from build123d import *

# Parameters (mm, degrees)
SKETCH1_W            = 30
SKETCH1_H            = 105
BOSS_EXTRUDE1_DEPTH  = 4
SKETCH2_W            = 30
SKETCH2_H            = 12
SKETCH2_R            = 1.8
BOSS_EXTRUDE2_DEPTH  = 4
SKETCH3_W            = 7
SKETCH3_H            = 16
CUT_EXTRUDE1_DEPTH   = 110.494292089
BOSS_EXTRUDE3_DEPTH  = 4
BOSS_EXTRUDE4_START  = -30
BOSS_EXTRUDE4_DEPTH  = 4
SKETCH5_W            = 30
SKETCH5_H            = 41
BOSS_EXTRUDE5_DEPTH  = 4
SKETCH6_W            = 30
SKETCH6_H            = 135
BOSS_EXTRUDE6_DEPTH  = 4
SKETCH7_W            = 30
SKETCH7_H            = 8.5
BOSS_EXTRUDE7_DEPTH  = 4
FILLET1_R            = 1.1
SKETCH10_W           = 2.15
SKETCH10_H           = 4
SKETCH11_W           = 8
SKETCH11_H           = 8.5
CUT_EXTRUDE2_DEPTH   = 16
SKETCH14_W           = 1.8
SKETCH14_H           = 30
BOSS_EXTRUDE8_DEPTH  = 1
SKETCH16_W           = 3.4
SKETCH16_H           = 4
BOSS_EXTRUDE10_DEPTH = 1
BOSS_EXTRUDE9_START  = -30
BOSS_EXTRUDE9_DEPTH  = 1
SKETCH17_W           = 3.4
SKETCH17_H           = 4
BOSS_EXTRUDE11_DEPTH = 1
CHAMFER1_SIZE        = 3
FILLET2_R            = 2


with BuildPart() as part:
    # Sketch1 → Boss-Extrude1 (new body)
    with BuildSketch(Plane.XY):
        with Locations((15, 52.5)):
            Rectangle(SKETCH1_W, SKETCH1_H)
    extrude(amount=BOSS_EXTRUDE1_DEPTH)

    # Sketch2 → Boss-Extrude2 (add)
    with BuildSketch(Plane.XZ):
        with Locations((15, 6)):
            Rectangle(SKETCH2_W, SKETCH2_H)
        with Locations((15, 5)):
            Circle(SKETCH2_R, mode=Mode.SUBTRACT)
    extrude(amount=-BOSS_EXTRUDE2_DEPTH)

    # Sketch3 → Cut-Extrude1 (cut, through all)
    with BuildSketch(Plane.XY.offset(4)):
        with Locations((15, 12)):
            Rectangle(SKETCH3_W, SKETCH3_H)
    extrude(amount=-CUT_EXTRUDE1_DEPTH, mode=Mode.SUBTRACT)

    # Sketch4 → Boss-Extrude3 (add)
    with BuildSketch(Plane.ZY):
        Polygon((12, 4), (0, 34), (0, 4), align=None)
    extrude(amount=-BOSS_EXTRUDE3_DEPTH)

    # Sketch4<2> → Boss-Extrude4 (add)
    with BuildSketch(Plane.ZY.offset(BOSS_EXTRUDE4_START)):
        Polygon((12, 4), (0, 34), (0, 4), align=None)
    extrude(amount=BOSS_EXTRUDE4_DEPTH)

    # Sketch5 → Boss-Extrude5 (add)
    with BuildSketch(Plane(origin=(0, 105, 0), x_dir=(1, 0, 0), z_dir=(0, 1, 0))):
        with Locations((15, 16.5)):
            Rectangle(SKETCH5_W, SKETCH5_H)
    extrude(amount=BOSS_EXTRUDE5_DEPTH)

    # Sketch6 → Boss-Extrude6 (add)
    with BuildSketch(Plane(origin=(0, 0, -37), x_dir=(-1, 0, 0), z_dir=(0, 0, -1))):
        with Locations((-15, 41.5)):
            Rectangle(SKETCH6_W, SKETCH6_H)
    extrude(amount=-BOSS_EXTRUDE6_DEPTH)

    # Sketch7 → Boss-Extrude7 (add)
    with BuildSketch(Plane.XZ.offset(26)):
        with Locations((15, -37.25)):
            Rectangle(SKETCH7_W, SKETCH7_H)
    extrude(amount=-BOSS_EXTRUDE7_DEPTH)

    # Fillet1
    fillet1_edges = [part.edges().sort_by_distance(p)[0] for p in [
        (0, -24, -41.5),
        (30, -24, -41.5),
    ]]
    fillet(fillet1_edges, radius=FILLET1_R)

    # Sketch10 → Ø4.3 (4.3) Diameter Hole1 (revolve, cut)
    with BuildSketch(Plane(origin=(15, -22, -37.5), x_dir=(0, 0, 1), z_dir=(1, 0, 0))):
        with Locations((1.075, 2)):
            Rectangle(SKETCH10_W, SKETCH10_H)
    revolve(axis=Axis((15, -15.65, -37.5), (0, -1, 0)), mode=Mode.SUBTRACT)

    # Sketch11 → Cut-Extrude2 (cut)
    with BuildSketch(Plane(origin=(0, -22, 0), x_dir=(1, 0, 0), z_dir=(0, 1, 0))):
        with Locations((15, 37.25)):
            Rectangle(SKETCH11_W, SKETCH11_H)
    extrude(amount=CUT_EXTRUDE2_DEPTH, mode=Mode.SUBTRACT)

    # Sketch14 → Ø3.6 (3.6) Diameter Hole1 (revolve, cut)
    with BuildSketch(Plane(origin=(15, 4, 5), x_dir=(0, 0, 1), z_dir=(1, 0, 0))):
        with Locations((0.9, 15)):
            Rectangle(SKETCH14_W, SKETCH14_H)
    revolve(axis=Axis((15, 10.35, 5), (0, -1, 0)), mode=Mode.SUBTRACT)

    # Sketch15 → Boss-Extrude8 (add)
    with BuildSketch(Plane.ZY):
        Polygon((-37, 109), (4, 109), (4, 0), (-1.5, 0), (-1.5, 103.5), (-31.5, 103.5), (-31.5, -26), (-37, -26), align=None)
    extrude(amount=BOSS_EXTRUDE8_DEPTH)

    # Sketch16 → Boss-Extrude10 (add)
    with BuildSketch(Plane.ZY):
        Polygon((4, 24), (4, 0), (12, 0), (12, 4), align=None)
        with Locations((-38.7, -24)):
            Rectangle(SKETCH16_W, SKETCH16_H)
    extrude(amount=BOSS_EXTRUDE10_DEPTH)

    # Sketch15<2> → Boss-Extrude9 (add)
    with BuildSketch(Plane.ZY.offset(BOSS_EXTRUDE9_START)):
        Polygon((-37, 109), (4, 109), (4, 0), (-1.5, 0), (-1.5, 103.5), (-31.5, 103.5), (-31.5, -26), (-37, -26), align=None)
    extrude(amount=-BOSS_EXTRUDE9_DEPTH)

    # Sketch17 → Boss-Extrude11 (add)
    with BuildSketch(Plane(origin=(30, 0, 0), x_dir=(0, 0, -1), z_dir=(1, 0, 0))):
        Polygon((-12, 0), (-4, 0), (-4, 24), (-12, 4), align=None)
        with Locations((38.7, -24)):
            Rectangle(SKETCH17_W, SKETCH17_H)
    extrude(amount=BOSS_EXTRUDE11_DEPTH)

    # Chamfer1
    chamfer1_edges = [part.edges().sort_by_distance(p)[0] for p in [
        (15, 109, 4),
        (15, 109, -37),
    ]]
    chamfer(chamfer1_edges, length=CHAMFER1_SIZE)

    # Fillet2
    # the kernel refuses this fillet: 2 mm, written as the material it takes off along each edge
    with BuildSketch(Plane(origin=(-1, 111, 4), x_dir=(1, 0, 0), z_dir=(0, -1, 0))) as fillet2_piece_1_section:
        with BuildLine():
            CenterArc((FILLET2_R, -FILLET2_R), FILLET2_R, 90, 90)
            Line((0, -FILLET2_R), (0, 0))
            Line((0, 0), (FILLET2_R, 0))
        make_face()
    fillet2_piece_1 = extrude(amount=92, mode=Mode.PRIVATE)
    fillet2_piece_1 = split(fillet2_piece_1, bisect_by=Plane(origin=(-0.544012224, 62.136356158, -11.254542463), z_dir=(0, 0.3713906763541038, 0.9284766908852594)), keep=Keep.TOP, mode=Mode.PRIVATE)
    add(fillet2_piece_1, mode=Mode.SUBTRACT)
    with BuildSketch(Plane(origin=(31, 111, 4), x_dir=(-1, 0, 0), z_dir=(0, -1, 0))) as fillet2_piece_2_section:
        with BuildLine():
            CenterArc((FILLET2_R, FILLET2_R), FILLET2_R, 180, 90)
            Line((0, FILLET2_R), (0, 0))
            Line((0, 0), (FILLET2_R, 0))
        make_face()
    fillet2_piece_2 = extrude(amount=92, mode=Mode.PRIVATE)
    fillet2_piece_2 = split(fillet2_piece_2, bisect_by=Plane(origin=(30.544012224, 62.136356158, -11.254542463), z_dir=(0, 0.37139067635410367, 0.9284766908852594)), keep=Keep.TOP, mode=Mode.PRIVATE)
    add(fillet2_piece_2, mode=Mode.SUBTRACT)
    with BuildSketch(Plane(origin=(-1, 109, -39), x_dir=(0, -1, 0), z_dir=(0, 0, 1))) as fillet2_piece_3:
        with BuildLine():
            CenterArc((FILLET2_R, FILLET2_R), FILLET2_R, 180, 90)
            Line((0, FILLET2_R), (0, 0))
            Line((0, 0), (FILLET2_R, 0))
        make_face()
    extrude(amount=45, mode=Mode.SUBTRACT)
    with BuildSketch(Plane(origin=(31, 109, -39), x_dir=(0, -1, 0), z_dir=(0, 0, 1))) as fillet2_piece_4:
        with BuildLine():
            CenterArc((FILLET2_R, -FILLET2_R), FILLET2_R, 90, 90)
            Line((0, -FILLET2_R), (0, 0))
            Line((0, 0), (FILLET2_R, 0))
        make_face()
    extrude(amount=45, mode=Mode.SUBTRACT)
    with BuildSketch(Plane(origin=(-1, -22, -37), x_dir=(0, 0, 1), z_dir=(0, 1, 0))) as fillet2_piece_5:
        with BuildLine():
            CenterArc((FILLET2_R, FILLET2_R), FILLET2_R, 180, 90)
            Line((0, FILLET2_R), (0, 0))
            Line((0, 0), (FILLET2_R, 0))
        make_face()
    extrude(amount=133, mode=Mode.SUBTRACT)
    with BuildSketch(Plane(origin=(-1, 102.464466094, 7.535533906), x_dir=(0, -0.7071067811865476, -0.7071067811865476), z_dir=(0, 0.7071067811865476, -0.7071067811865476)), Plane(origin=(-1, 112.535533906, -30.464466094), x_dir=(0, -0.7071067811865476, 0.7071067811865476), z_dir=(0, -0.7071067811865476, -0.7071067811865476)), Plane(origin=(31, 102.464466094, 7.535533906), x_dir=(-1, 0, 0), z_dir=(0, 0.7071067811865476, -0.7071067811865476))) as fillet2_piece_6:
        with BuildLine():
            CenterArc((FILLET2_R, -FILLET2_R), FILLET2_R, 90, 90)
            Line((0, -FILLET2_R), (0, 0))
            Line((0, 0), (FILLET2_R, 0))
        make_face()
    extrude(amount=14.242640687, mode=Mode.SUBTRACT)
    with BuildSketch(Plane(origin=(31, -22, -37), x_dir=(0, 0, 1), z_dir=(0, 1, 0))) as fillet2_piece_7:
        with BuildLine():
            CenterArc((FILLET2_R, -FILLET2_R), FILLET2_R, 90, 90)
            Line((0, -FILLET2_R), (0, 0))
            Line((0, 0), (FILLET2_R, 0))
        make_face()
    extrude(amount=133, mode=Mode.SUBTRACT)
    with BuildSketch(Plane(origin=(31, 112.535533906, -30.464466094), x_dir=(0, -0.7071067811865476, 0.7071067811865476), z_dir=(0, -0.7071067811865476, -0.7071067811865476))) as fillet2_piece_8:
        with BuildLine():
            CenterArc((FILLET2_R, FILLET2_R), FILLET2_R, 180, 90)
            Line((0, FILLET2_R), (0, 0))
            Line((0, 0), (FILLET2_R, 0))
        make_face()
    extrude(amount=14.242640687, mode=Mode.SUBTRACT)


solid = part.part
Here's how the part is built. I have some questions about the finished solid (model axes, mm). A direction names the side the tool comes from. Coordinates: 2 decimals unless noted, no trailing zeros. Write each loop counter-clockwise with the first axis right and the second up, starting at its lowest first coordinate (ties: lowest second). Pieces come first, ordered by that corner, then holes. Notation, with made-up numbers: (31, 55.25) - (54, 55.25) arc R25 ccw to (54, 94.25) - close; hole circle Ø6 at (53, 26.25). An arc over 180 degrees is marked (long way). Use one line per item in the form item = value.
1) Suppose I cut it at C-C, the plane z = -3.5. Write out the boundary of the cut face in (x, y), plus the area to 3 significant figures.
Solved:
outline = (-1, 103.5) - (0, 103.5) - (0, 105) - (30, 105) - (30, 103.5) - (31, 103.5) - (31, 107) arc R2 ccw to (29, 109) - (1, 109) arc R2 ccw to (-1, 107) - close
area = 129 mm2
2) On a 3-axis mill with a long thin cutter (end or side, diameter ignored), from which of +Z, -Z, +X, -X, +Y, -Y can I reach the whole of each face in a straight line? I mean faces 1 (the flat face through (15, 40, -33)), 2 (the flat face through (15, -6, -35)), 3 (the flat face through (15, 4, 7)). Say none if no direction works.
Solved:
face_1 = -Y
face_2 = +Z, -Z
face_3 = +Z
3) Suppose I cut it at B-B, the plane x = 15. Write out the boundary of the cut face in (y, z), plus the area to 3 significant figures.
Solved:
outline = (-26, -41.5) - (-22, -41.5) - (-22, -39.65) - (-26, -39.65) - close; (-26, -35.35) - (-22, -35.35) - (-22, -33) - (-26, -33) - close; (-6, -37) - (106, -37) - (109, -34) - (109, 1) - (106, 4) - (20, 4) - (20, 0) - (105, 0) - (105, -33) - (-6, -33) - close; (0, 0) - (4, 0) - (4, 3.2) - (0, 3.2) - close; (0, 6.8) - (4, 6.8) - (4, 12) - (0, 12) - close
area = 989 mm2
4) Suppose I cut it at A-A, the plane y = 37.5. Write out the boundary of the cut face in (x, z), plus the area to 3 significant figures.
Solved:
outline = (-1, -35) arc R2 ccw to (1, -37) - (29, -37) arc R2 ccw to (31, -35) - (31, -31.5) - (30, -31.5) - (30, -33) - (0, -33) - (0, -31.5) - (-1, -31.5) - close; (-1, -1.5) - (0, -1.5) - (0, 0) - (30, 0) - (30, -1.5) - (31, -1.5) - (31, 2) arc R2 ccw to (29, 4) - (1, 4) arc R2 ccw to (-1, 2) - close
area = 259 mm2
5) I need wall thicknesses on line 1 (Z direction, x = 15, y = 1); line 2 (Z direction, x = 20.5, y = 18.5); line 3 (X direction, y = -24.75, z = -37.5). Which ranges of each line are inside material? Lowest first, please.
Solved:
line_1 = -37 to -33, 0 to 3.2, 6.8 to 12
line_2 = -37 to -33, 0 to 4
line_3 = -1 to 12.85, 17.15 to 31
6) Suppose I cut it at D-D, the plane y = -17. Write out the boundary of the cut face in (x, z).
Solved:
outline = (-1, -35) arc R2 ccw to (1, -37) - (11, -37) - (11, -33) - (0, -33) - (0, -31.5) - (-1, -31.5) - close; (19, -37) - (29, -37) arc R2 ccw to (31, -35) - (31, -31.5) - (30, -31.5) - (30, -33) - (19, -33) - close
7) I'm going to push flat-ended pins straight in: P1, Ø2, axis at x = 17, z = -36, coming from the +Y side; P2, Ø0.8, axis at x = -0.5, y = -23, coming from the -Z side; P3, Ø0.5, axis at x = 30.5, y = 19.5, coming from the +Z side. Where does each tip first touch, or does it pass through?
Solved:
P1 = 108
P2 = -40.4
P3 = 5.9
8) Thinking about a two-plate mould opening in Z: for faces 4 (the cylindrical face through (13.87, 1.97, 3.6)), 5 (the flat face through (11.5, 12, 2)), 6 (the flat face through (15, 56, 4)), which applies, released by +Z, released by -Z, zero draft, split by the parting line, or undercut?
Solved:
face_4 = undercut
face_5 = zero draft
face_6 = released by +Z
